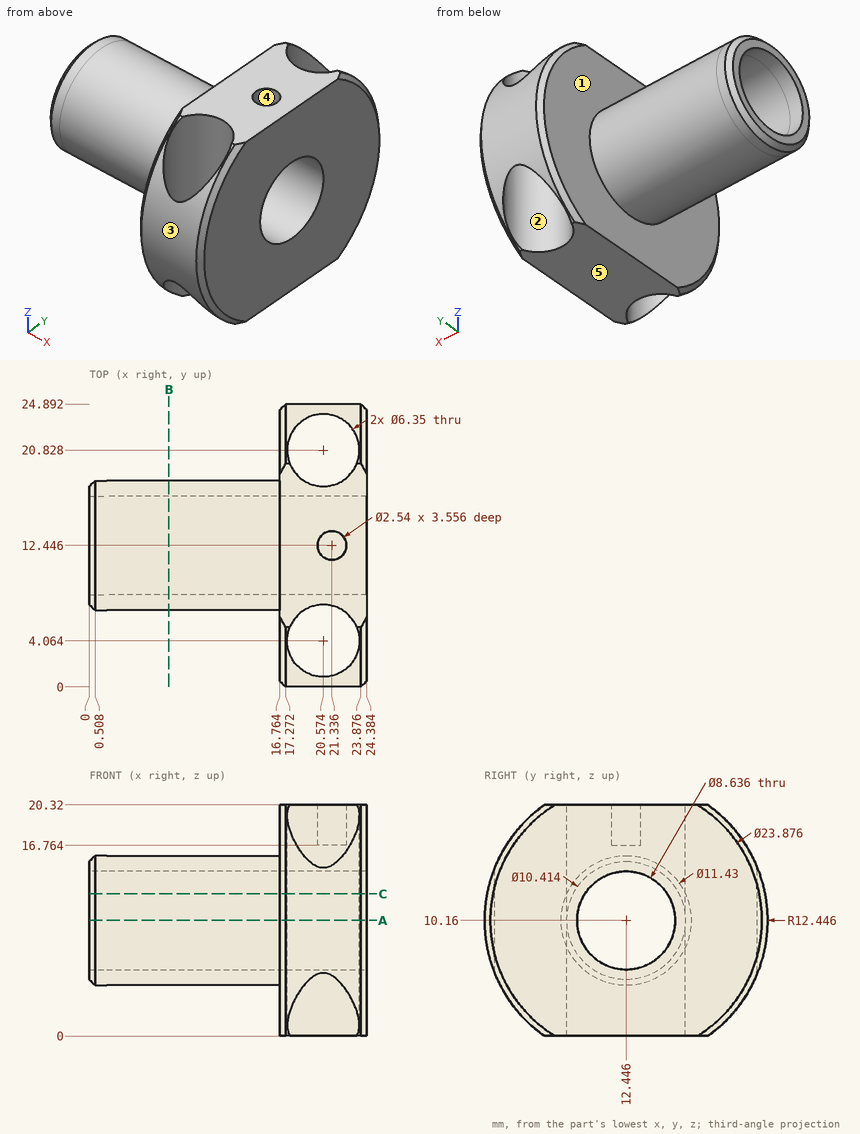
Could you check a few things on this drawing? It's one solid part, dimensions in mm from its lowest x, y, z. A direction names the side the tool comes from. Coordinates: 2 decimals unless noted, no trailing zeros. Write each loop counter-clockwise with the first axis right and the second up, starting at its lowest first coordinate (ties: lowest second). Pieces come first, ordered by that corner, then holes. Notation, with made-up numbers: (33.5, -21) - (42.5, -21) arc R24 cw to (42.5, 16) - close; hole circle Ø11 at (-5, -28.5). An arc over 180 degrees is marked (long way). Use one line per item in the form item = value.
1) I need wall thicknesses on line 1 (Y direction, x = 0.75, z = 10.16); line 2 (Y direction, x = 20, z = 10.75); line 3 (Y direction, x = 14.75, z = 13). Which ranges of each line are inside material? Lowest first, please.
Solved:
line_1 = 6.73 to 8.13, 16.76 to 18.16
line_2 = 0.01 to 0.94, 7.19 to 8.17, 16.72 to 17.71, 23.95 to 24.88
line_3 = 7.49 to 9.19, 15.7 to 17.41
2) I'm going to push flat-ended pins straight in: P1, Ø8, axis at y = 2.5, z = 4, coming from the -X side; P2, Ø5, axis at x = 10, z = 17, coming from the -Y side; P3, Ø0.8, axis at x = 21, y = 12.5, coming from the +Z side. Where does each tip first touch, or does it pass through?
Solved:
P1 = 16.76
P2 = 8.73
P3 = 16.76
3) Suppose I cut it at C-C, the plane z = 12.5. Give the number of separate pieces and of enclosed holes in the cut face, plus the area to 3 significant figures.
Solved:
separate_pieces = 2
enclosed_holes = 2
area = 120 mm2
4) Thinking about a two-plate mould opening in Y: for the marked faces 1, 2 and 3, which applies, released by +Y, released by -Y, zero draft, split by the parting line, or undercut?
Solved:
face_1 = zero draft
face_2 = undercut
face_3 = released by -Y
5) Suppose I cut it at B-B, the plane x = 7. Write out the boundary of the cut face in (y, z) (3 decimals).
Solved:
outline = circle Ø11.43 at (12.446, 10.16); hole circle Ø8.636 at (12.446, 10.16)
6) Suppose I cut it at A-A, the plane z = 10.16. Write out the boundary of the cut face in (x, y) (3 decimals), plus the area to 3 significant figures.
Solved:
outline = (0, 7.239) - (0.508, 6.731) - (16.764, 6.731) - (16.764, 0.508) - (17.272, 0) - (23.876, 0) - (24.384, 0.508) - (24.384, 8.128) - (0, 8.128) - close; (0, 16.764) - (24.384, 16.764) - (24.384, 24.384) - (23.876, 24.892) - (17.272, 24.892) - (16.764, 24.384) - (16.764, 18.161) - (0.508, 18.161) - (0, 17.653) - close; hole circle Ø6.35 at (20.574, 4.064); hole circle Ø6.35 at (20.574, 20.828)
area = 107 mm2
7) On a 3-axis mill with a long thin cutter (end or side, diameter ignored), from which of +Z, -Z, +X, -X, +Y, -Y can I reach the whole of each face in a straight line? I mean the marked faces 4 and 5. Say none if no direction works.
Solved:
face_4 = +Z
face_5 = -Z, +X, -X, +Y, -Y
